Can you work these out from the model? Positions are in its coordinate system, mm. A direction names the side the tool comes from. Give positions to 0.01 mm unless a question says otherwise; leave off trailing zeros. Loops run counter-clockwise (first coordinate to the right, second up) from the corner with the lowest first, then second, coordinate; pieces in that order, holes last. Notation, with made-up numbers: (-2.75, 58.5) - (52.25, 58.5) arc R20 cw to (52.25, 68.5) - close; hole circle Ø5 at (-30.5, -30). An arc over 180 degrees is marked (long way). Answer as a JSON object with one key per item and string values. Group by question number.
Item 1: Thinking about a two-plate mould opening in Z: for faces 1 (the flat face through (157.924, 138, -1)), 2 (the flat face through (-30.925, 138, -1)), 3 (the flat face through (-220.662, 138, -1)), which applies, pulls with the +Z half, pulls with the -Z half, needs draft (parallel to the pull), parting line crosses it, or undercut?
Item 2: Which directions (+Z, -Z, +X, -X, +Y, -Y) give clear straight access to the entire face, cutting with the end or side of a thin tool? Please do faces 4 (the flat face through (-48, 138, 64.287)), 5 (the flat face through (32, 0, 10)).
Item 3: Suppose I cut it at B-B on y = 108.5. Count the separate pieces of the cut face and the enclosed holes in it, and give its area (3 significant figures).
Item 4: Suppose I cut it at A-A on x = -46.5. Write out the boundary of the cut face in (y, z) (3 decimals).
Item 5: Please list where this line runs through material, in increasing order: L1, parallel to Z at x = 135.5, y = 250.5 (3 decimals).
from build123d import *

# Parameters (mm, degrees)
F0_W     = 441.325
F0_H     = 133.35
F0_W_2   = 30.099
F0_H_2   = 128.5748
F1_DEPTH = 279.4


with BuildPart() as f1:
    # F0 (on Front) → F1 (new body)
    with BuildSketch(Plane.XZ):
        Rectangle(F0_W, F0_H)
        with Locations((-174.625, -2e-06)):
            Rectangle(F0_W_2, F0_H_2, mode=Mode.SUBTRACT)
        with Locations((-142.875, -2e-06)):
            Rectangle(F0_W_2, F0_H_2, mode=Mode.SUBTRACT)
        with Locations((-111.125, -2e-06)):
            Rectangle(F0_W_2, F0_H_2, mode=Mode.SUBTRACT)
        with Locations((-79.375, -2e-06)):
            Rectangle(F0_W_2, F0_H_2, mode=Mode.SUBTRACT)
        with Locations((-47.625, -2e-06)):
            Rectangle(F0_W_2, F0_H_2, mode=Mode.SUBTRACT)
        with Locations((-15.875, -2e-06)):
            Rectangle(F0_W_2, F0_H_2, mode=Mode.SUBTRACT)
        with Locations((15.875, -2e-06)):
            Rectangle(F0_W_2, F0_H_2, mode=Mode.SUBTRACT)
        with Locations((47.625, -2e-06)):
            Rectangle(F0_W_2, F0_H_2, mode=Mode.SUBTRACT)
        with Locations((79.375, -2e-06)):
            Rectangle(F0_W_2, F0_H_2, mode=Mode.SUBTRACT)
        with Locations((111.125, -2e-06)):
            Rectangle(F0_W_2, F0_H_2, mode=Mode.SUBTRACT)
        with Locations((142.875, -2e-06)):
            Rectangle(F0_W_2, F0_H_2, mode=Mode.SUBTRACT)
        with Locations((174.625, -2e-06)):
            Rectangle(F0_W_2, F0_H_2, mode=Mode.SUBTRACT)
    extrude(amount=-F1_DEPTH)


solid = f1.part
Worked out:
{
 "1": {"face 1": "undercut", "face 2": "undercut", "face 3": "needs draft"},
 "2": {"face 4": "+Y, -Y", "face 5": "+Z, -Z, +X, -X, -Y"},
 "3": {"separate pieces": "1", "enclosed holes": "12", "area": "12,400 mm2"},
 "4": {"outline": "(0, -66.675) - (279.4, -66.675) - (279.4, -64.287) - (0, -64.287) - close; (0, 64.287) - (279.4, 64.287) - (279.4, 66.675) - (0, 66.675) - close"},
 "5": {"L1": "z = -66.675 to -64.287, 64.287 to 66.675"}
}
